Study the drawing (mm; zero at the part's minimum x, y, z) and answer. Coordinates: 2 decimals unless noted, no trailing zeros. Order: outer loops, then holes, each group sorted by start corner. A loop starts at its lowest first (then second) coordinate and runs counter-clockwise, first axis right, second up. Notation, with made-up numbers: M 51.25,1.5 L 89.25,1.5 A23 ccw 89.25,28.5 Z; hole C 26,83 d3. An arc over 180 degrees is marked long. One line per item, written item: value. Start each with the question number.
Q1. The part is cut by section D-D on y = 16. Give the vertices of the cut face in (x, z), then the cut area to 3 significant figures.
Q2. The part is cut by section A-A on x = 114.3. Give the vertices of the cut face in (y, z) (1 decimal).
Q3. The part is cut by section B-B on y = 114.3. Give the vertices of the cut face in (x, z).
Q4. Straight lines are drawn through the part: line 1 along Y through (x, z) = (114.3, 2.8) (1 decimal); line 2 along Y through (x, z) = (136.5, 2.3); line 3 along Y through (x, z) = (93, 2.05) (1 decimal). For each, find the intervals that lie inside material, in ascending order. Write a range as [from, to].
Q5. Each of these flat-tipped pins is pushed along its axis until it touches: pin 1 Ø2 at (y, z) = (129.5, 2.5) entering from -X (1 decimal); pin 2 Ø1 at (y, z) = (105, 1) entering from -X; pin 3 Ø2 at (y, z) = (94, 2.5) entering from +X. Where does it stop, or does it pass through?
Q6. The part is cut by section C-C on z = 1.55. Give the vertices of the cut face in (x, y) (1 decimal).
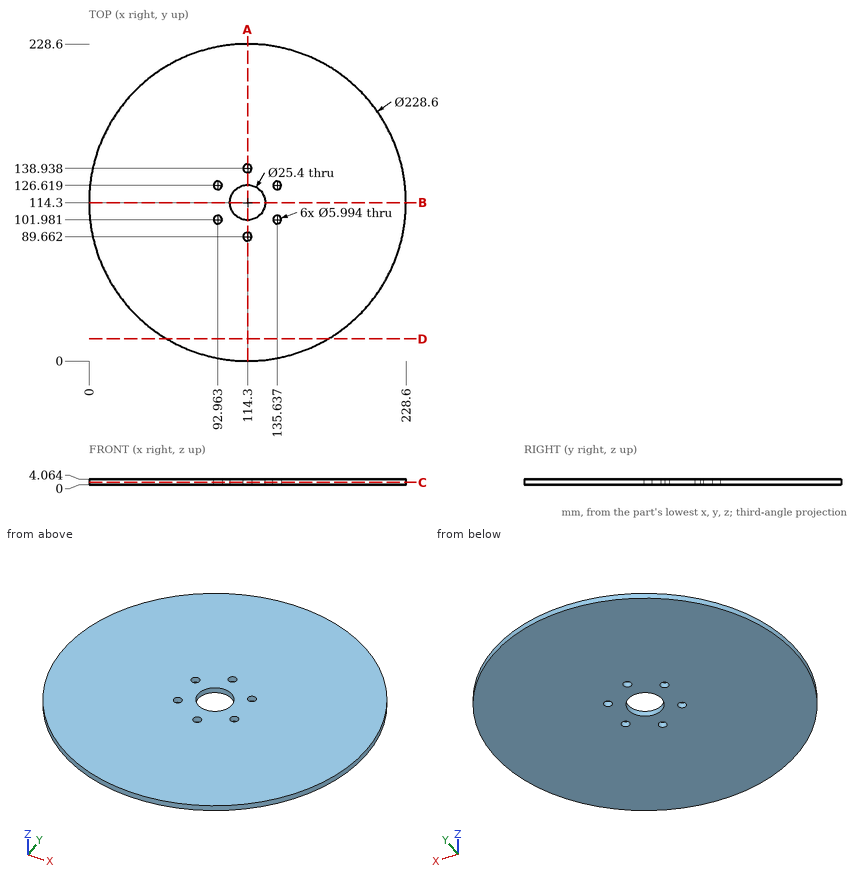
Output:
1. outline: M 55.98,0 L 172.62,0 L 172.62,4.06 L 55.98,4.06 Z
1. area: 474 mm^2
2. outline: M 0,0 L 86.7,0 L 86.7,4.1 L 0,4.1 Z; M 92.7,0 L 101.6,0 L 101.6,4.1 L 92.7,4.1 Z; M 127,0 L 135.9,0 L 135.9,4.1 L 127,4.1 Z; M 141.9,0 L 228.6,0 L 228.6,4.1 L 141.9,4.1 Z
3. outline: M 0,0 L 101.6,0 L 101.6,4.06 L 0,4.06 Z; M 127,0 L 228.6,0 L 228.6,4.06 L 127,4.06 Z
4. line 1: y = [0, 86.7], [92.7, 101.6], [127, 135.9], [141.9, 228.6]
4. line 2: y = [2.18, 99.11], [104.85, 123.75], [129.49, 226.42]
4. line 3: y = [2, 99], [105, 123.6], [129.6, 226.6]
5. pin 1: stops at x = 0.9
5. pin 2: stops at x = 0.34
5. pin 3: stops at x = 226.96
6. outline: C 114.3,114.3 d228.6; hole C 93,102 d6; hole C 93,126.6 d6; hole C 114.3,114.3 d25.4; hole C 114.3,89.7 d6; hole C 114.3,138.9 d6; hole C 135.6,102 d6; hole C 135.6,126.6 d6
